```python
from build123d import *

# Parameters (mm, degrees)
EXTRUDE_2_DEPTH = 10


with BuildPart() as part:
    # Эскиз2 → Бобышка-Вытянуть2 (new body)
    with BuildSketch(Plane(origin=(0, 0, 0), x_dir=(1, 0, 0), z_dir=(0, 1, 0))):
        with BuildLine():
            Line((-12.853030774, -2.577511611), (-12.853030774, -4.077511611))
            Line((-12.853030774, -4.077511611), (-14.353030774, -4.077511611))
            Line((-14.353030774, -4.077511611), (-14.353030774, -2.927511611))
            ThreePointArc((-14.353030774, -2.927511611), (-14.528030774, -2.624402719), (-14.878030774, -2.624402719))
            Line((-14.878030774, -2.624402719), (-20.16700352, -5.677992558))
            ThreePointArc((-20.16700352, -5.677992558), (-20.516447889, -6.521625894), (-19.79200352, -7.077511611))
            Line((-19.79200352, -7.077511611), (-7.73171043, -7.077511611))
            Line((-7.73171043, -7.077511611), (2.26828957, 2.922488389))
            Line((2.26828957, 2.922488389), (6.146969226, 2.922488389))
            Line((6.146969226, 2.922488389), (6.146969226, -7.577511611))
            Line((6.146969226, -7.577511611), (10.646969226, -7.577511611))
            Line((10.646969226, -7.577511611), (10.646969226, -6.077511611))
            Line((10.646969226, -6.077511611), (7.646969226, -6.077511611))
            Line((7.646969226, -6.077511611), (7.646969226, -0.077511611))
            Line((7.646969226, -0.077511611), (9.146969226, -0.077511611))
            Line((9.146969226, -0.077511611), (9.146969226, 5.285737044))
            Line((9.146969226, 5.285737044), (4.146969226, 8.172488389))
            Line((4.146969226, 8.172488389), (4.146969226, 5.922488389))
            Line((4.146969226, 5.922488389), (3.146969226, 5.922488389))
            Line((3.146969226, 5.922488389), (-6.045418929, -3.269899766))
            ThreePointArc((-6.045418929, -3.269899766), (-6.568677947, -3.486640748), (-7.091936965, -3.269899766))
            Line((-7.091936965, -3.269899766), (-7.106079101, -3.25575763))
            ThreePointArc((-7.106079101, -3.25575763), (-7.322820083, -2.732498612), (-7.106079101, -2.209239594))
            Line((-7.106079101, -2.209239594), (3.146969226, 8.043808733))
            Line((3.146969226, 8.043808733), (3.146969226, 40.922488389))
            Line((3.146969226, 40.922488389), (4.146969226, 40.922488389))
            Line((4.146969226, 40.922488389), (7.496211631, 37.573245985))
            Line((7.496211631, 37.573245985), (9.617531975, 37.573245985))
            Line((9.617531975, 37.573245985), (9.617531975, 39.694566328))
            Line((9.617531975, 39.694566328), (-3.110390087, 52.422488389))
            Line((-3.110390087, 52.422488389), (-16.353030774, 52.422488389))
            Line((-16.353030774, 52.422488389), (-16.353030774, 49.422488389))
            Line((-16.353030774, 49.422488389), (-14.353030774, 49.422488389))
            Line((-14.353030774, 49.422488389), (-14.353030774, 50.922488389))
            Line((-14.353030774, 50.922488389), (-12.853030774, 50.922488389))
            Line((-12.853030774, 50.922488389), (-12.853030774, 49.422488389))
            Line((-12.853030774, 49.422488389), (-4.353030774, 49.422488389))
            Line((-4.353030774, 49.422488389), (0.146969226, 44.922488389))
            Line((0.146969226, 44.922488389), (0.146969226, 9.28644942))
            Line((0.146969226, 9.28644942), (-11.716991804, -2.577511611))
            Line((-11.716991804, -2.577511611), (-12.853030774, -2.577511611))
        make_face()
    extrude(amount=EXTRUDE_2_DEPTH)


solid = part.part
```
Design review of the part built by this model. Coordinates are the model's own, in mm. A direction names the side the tool comes from. Round coordinates to 2 decimals unless told otherwise and drop trailing zeros. Write each loop counter-clockwise with the first axis right and the second up, starting at its lowest first coordinate (ties: lowest second). Pieces come first, ordered by that corner, then holes. Notation, with made-up numbers: (4.25, 33.5) -> (55.25, 33.5) arc R26 cw to (55.25, 57.5) -> close; hole circle Ø8 at (67, -8). An arc over 180 degrees is marked (long way). Write item = value, one per line. Start each with the question number.
1) Tool access review of faces 4 (the face through (8, 5, 7.578)), 5 (the face through (7.647, 5, 3)), 6 (the face through (-6.561, 4.93, 3.487)), 7 (the face through (-2.13, 4.93, -47.2)), 8 (the face through (-16.353, 5, -51)): name each direction out of +Z, -Z, +X, -X, +Y, -Y from which nothing blocks a thin tool from reaching the whole face with its end or side.
2) Take a section at A-A, the plane x = -0.5. State the section outline as (y, z) points.
3) Clearance check with flat-ended pins moving along their axes: pin 1 (2 mm diameter, centred on x = 6.5, y = 7, fed in from -Z); pin 2 (1 mm diameter, centred on x = 2.5, z = -36.5, fed in from -Y); pin 3 (1.2 mm diameter, centred on y = 4.5, z = -50.5, fed in from +X); pin 4 (0.6 mm diameter, centred on y = 5.5, z = -39, fed in from +X). State where each tip first meets the part, or that it passes through.
4) Take a section at B-B, the plane z = -34. State the section outline as (x, y) points.
5) Wall thickness on probe 1 along Z at (x, y) = (-5, 5); probe 2 along Z at (x, y) = (-4, 3.25); probe 3 along Z at (x, y) = (7, 3): over which ranges is each line inside the solid? List them lowest first. Write a range as from..to.
6) Mouldability with a two-part tool opening along Z and no side actions: class faces 1 (the face through (9.618, 5, -39)), 2 (the face through (4, 5, -2.922)), 3 (the face through (-14.353, 5, -50)) as +Z half, -Z half, draft (parallel to the pull), parting line (faces both ways), or undercut.
7) Take a section at C-C, the plane z = -47.5. State the section outline as (x, y) points, plus the area to 3 significant figures.
Results list:
q1.face_4 = +Z, +X, -X, +Y, -Y
q1.face_5 = +X, +Y, -Y
q1.face_6 = +Y, -Y
q1.face_7 = -X, +Y, -Y
q1.face_8 = -Z, -X, +Y, -Y
q2.outline = (0, -49.81) -> (10, -49.81) -> (10, -45.57) -> (0, -45.57) -> close; (0, -8.64) -> (10, -8.64) -> (10, -4.4) -> (0, -4.4) -> close; (0, -2.28) -> (10, -2.28) -> (10, -0.15) -> (0, -0.15) -> close
q3.pin_1 = -43.81
q3.pin_2 = 0
q3.pin_3 = -0.59
q3.pin_4 = 9.62
q4.outline = (0.15, 0) -> (3.15, 0) -> (3.15, 10) -> (0.15, 10) -> close
q5.probe_1 = -52.42..-49.42, -4.14..0.1, 2.22..4.35
q5.probe_2 = -52.42..-49.07, -5.14..-0.9, 1.22..3.35
q5.probe_3 = -42.31..-38.07, -6.53..7.58
q6.face_1 = draft
q6.face_2 = +Z half
q6.face_3 = undercut
q7.outline = (-2.43, 0) -> (1.81, 0) -> (1.81, 10) -> (-2.43, 10) -> close
q7.area = 42.4 mm²
